```python
from build123d import *

# Parameters (mm, degrees)
SKETCH1_W           = 40
SKETCH1_H           = 40
BOSS_EXTRUDE1_DEPTH = 5
BOSS_EXTRUDE2_START = 10
BOSS_EXTRUDE2_DEPTH = 20
CUT_EXTRUDE1_START  = -3
CUT_EXTRUDE1_DEPTH  = 5
CUT_EXTRUDE2_START  = -12
CUT_EXTRUDE2_DEPTH  = 5


with BuildPart() as part:
    # Sketch1 → Boss-Extrude1 (new body)
    with BuildSketch(Plane.XY):
        Rectangle(SKETCH1_W, SKETCH1_H)
    extrude(amount=BOSS_EXTRUDE1_DEPTH)

    # Sketch2 → Boss-Extrude2 (add)
    with BuildSketch(Plane(origin=(0, 0, 0), x_dir=(1, 0, 0), z_dir=(0, 1, 0)).offset(BOSS_EXTRUDE2_START)):
        with BuildLine():
            Line((10, -5), (-10, -5))
            Line((-10, -5), (-10, -20))
            ThreePointArc((-10, -20), (0, -30), (10, -20))
            Line((10, -20), (10, -5))
        make_face()
    extrude(amount=-BOSS_EXTRUDE2_DEPTH)

    # Sketch3 → Cut-Extrude1 (cut)
    with BuildSketch(Plane(origin=(0, 10, 0), x_dir=(1, 0, 0), z_dir=(0, 1, 0)).offset(CUT_EXTRUDE1_START)):
        with BuildLine():
            Line((10, -20), (10, -5))
            Line((10, -5), (-10, -5))
            Line((-10, -5), (-10, -20))
            ThreePointArc((-10, -20), (0, -30), (10, -20))
        make_face()
    extrude(amount=-CUT_EXTRUDE1_DEPTH, mode=Mode.SUBTRACT)

    # Sketch4 → Cut-Extrude2 (cut)
    with BuildSketch(Plane(origin=(0, 10, 0), x_dir=(1, 0, 0), z_dir=(0, 1, 0)).offset(CUT_EXTRUDE2_START)):
        with BuildLine():
            Line((10, -20), (10, -5))
            Line((10, -5), (-10, -5))
            Line((-10, -5), (-10, -20))
            ThreePointArc((-10, -20), (0, -30), (10, -20))
        make_face()
    extrude(amount=-CUT_EXTRUDE2_DEPTH, mode=Mode.SUBTRACT)


solid = part.part
```
The listing builds one solid part. Answer for the finished solid, in the listing's coordinates (mm). A direction names the side the tool comes from. Coordinates: 2 decimals unless noted, no trailing zeros. Write each loop counter-clockwise with the first axis right and the second up, starting at its lowest first coordinate (ties: lowest second). Pieces come first, ordered by that corner, then holes. Notation, with made-up numbers: (-10.75, -11.5) -> (22.25, -11.5) arc R29 cw to (22.25, 15.5) -> close; hole circle Ø3 at (-31, -10). An arc over 180 degrees is marked (long way). Write each question's results on one line, items separated by ' | '. Start each with the question number.
1) A cutting plane is placed at D-D (x = 13). Determine the outline of the cut face in (y, z), then the cut area to 3 significant figures.
2) For a pull along Y with two mould halves and no side action, classify faces 1 (the flat face through (0, -7, 17)), 2 (the flat face through (0, -20, 2)), 3 (the flat face through (0, 7, 17)), 4 (the flat face through (20, 0, 2)) as +Y half, -Y half, draft (parallel to the pull), parting line (faces both ways), or undercut.
3) A cutting plane is placed at C-C (y = -8). Determine the outline of the cut face in (x, z), then the cut area to 3 significant figures.
4) A cutting plane is placed at B-B (x = 0). Determine the outline of the cut face in (y, z), then the cut area to 3 significant figures.
5) A cutting plane is placed at A-A (z = 15). Determine the outline of the cut face in (x, y).
6) Flat-ended cylindrical pins translate along their axes: pin 1 Ø16 at (x, z) = (0, 16) entering from -Y; pin 2 Ø1.5 at (y, z) = (9, 11.5) entering from +X; pin 3 Ø3.5 at (y, z) = (-9, 15.5) entering from -X. Find the tip coordinate at first contact, or state that the pin passes through.
7) Straight lines are drawn through the part: probe 1 along Y at (x, z) = (3, 8.5); probe 2 along Z at (x, y) = (4, -15); probe 3 along X at (y, z) = (9, 25). For each, find the intervals that lie inside material, in ascending order.
8) A tool of negligible diameter and unlimited length cuts with its end or side. For faces 5 (the flat face through (-10, 0, 12)), 6 (the flat face through (10, -8, 13)), 7 (the flat face through (0, -10, 17)), 8 (the flat face through (0, 10, 17)), from which of +Z, -Z, +X, -X, +Y, -Y can it reach the whole face along a straight path? Write none if from no direction.
Values follow:
1) outline: (-20, 0) -> (20, 0) -> (20, 5) -> (-20, 5) -> close | area: 200 mm²
2) face 1: undercut | face 2: -Y half | face 3: undercut | face 4: draft
3) outline: (-20, 0) -> (20, 0) -> (20, 5) -> (10, 5) -> (10, 20) arc R10 ccw to (-10, 20) -> (-10, 5) -> (-20, 5) -> close | area: 657 mm²
4) outline: (-20, 0) -> (20, 0) -> (20, 5) -> (10, 5) -> (10, 30) -> (7, 30) -> (7, 5) -> (2, 5) -> (2, 30) -> (-2, 30) -> (-2, 5) -> (-7, 5) -> (-7, 30) -> (-10, 30) -> (-10, 5) -> (-20, 5) -> close | area: 450 mm²
5) outline: (-10, -10) -> (10, -10) -> (10, -7) -> (-10, -7) -> close; (-10, -2) -> (10, -2) -> (10, 2) -> (-10, 2) -> close; (-10, 7) -> (10, 7) -> (10, 10) -> (-10, 10) -> close
6) pin 1: y = -10 | pin 2: x = 10 | pin 3: x = -10
7) probe 1: -10 to -7, -2 to 2, 7 to 10 | probe 2: 0 to 5 | probe 3: -8.66 to 8.66
8) face 5: +Z, -X, +Y, -Y | face 6: +Z, +X, +Y, -Y | face 7: +Z, +X, -X, -Y | face 8: +Z, +X, -X, +Y
